Geometry: see drawing. Coordinates: mm, zero at the bounding-box minimum. A direction names the side the tool comes from. Coordinates: 2 decimals unless noted, no trailing zeros. Write each loop counter-clockwise with the first axis right and the second up, starting at its lowest first coordinate (ties: lowest second). Pieces come first, ordered by that corner, then holes. Notation, with made-up numbers: M 75.5,9 L 112.5,9 A32 cw 112.5,44 Z; hole C 68.5,41 d3. An arc over 180 degrees is marked long. Write item = value, one per line. Start each with the question number.
1. Pull-direction query (X, two-part tool) for the marked faces 3 and 4; classes: pulls with the +X half, pulls with the -X half, needs draft (parallel to the pull), parting line crosses it, or undercut.
2. Section query A-A (y = 15). Output: boundary loops of the cut face in (x, z).
3. Access query for the marked faces 1 and 2. Directions: +Z, -Z, +X, -X, +Y, -Y. A direction counts if a zero-diameter tool reaches every point of the face in a straight line with its end or side. Return the directions, or none.
4. Section query B-B (z = 24). Output: boundary loops of the cut face in (x, y), then the cut area to 3 significant figures.
5. Section query C-C (x = 49). Output: boundary loops of the cut face in (y, z).
6. Section query D-D (z = 47.5). Output: boundary loops of the cut face in (x, y).
7. Line query: line 1 along X through (y, z) = (16.5, 8); line 2 along Y through (x, z) = (75, 20); line 3 along Z through (x, y) = (63.5, 2). Output: solid intervals per line, ascending.
8. Pin query (flat end, axial travel): pin 1 Ø1.5 at (x, y) = (6, 21) entering from +Z; pin 2 Ø6 at (x, z) = (29.5, 41) entering from -Y; pin 3 Ø1.5 at (x, y) = (72, 20.5) entering from -Z. Return the tip coordinate at first contact, or that it passes through.
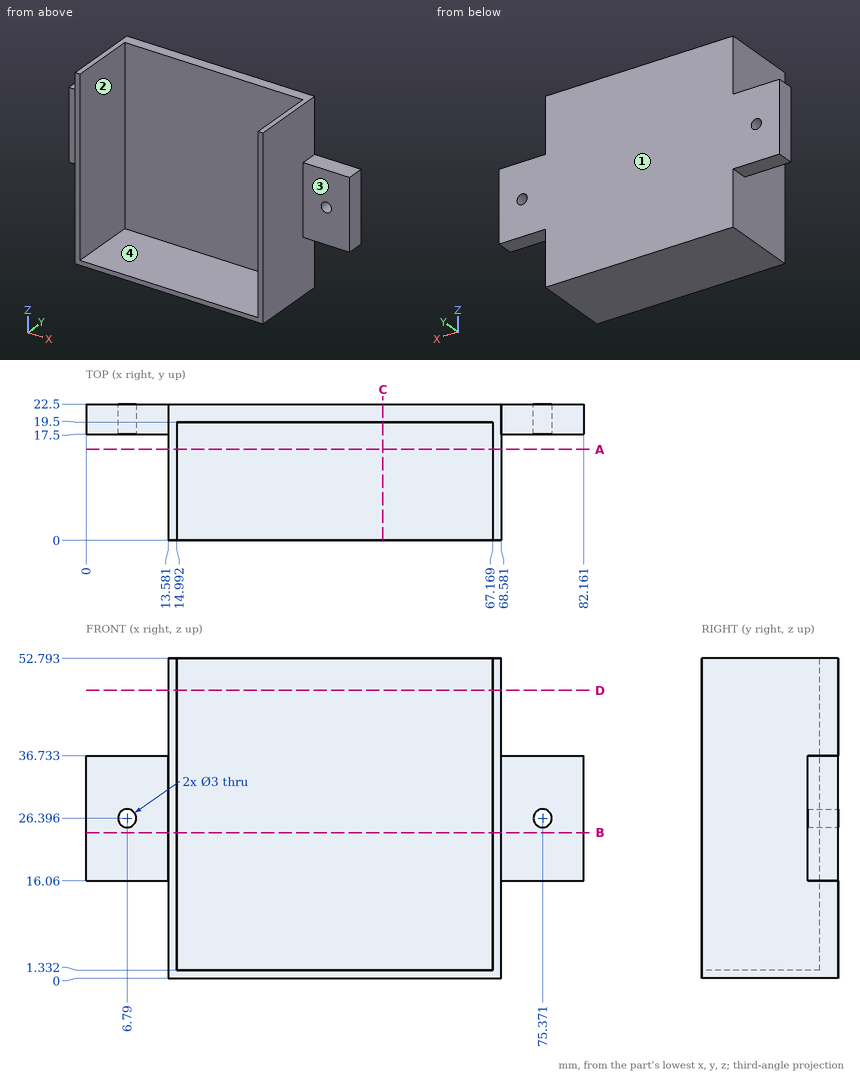
Results are:
q1.face_3 = needs draft
q1.face_4 = undercut
q2.outline = M 13.58,0 L 68.58,0 L 68.58,52.79 L 67.17,52.79 L 67.17,1.33 L 14.99,1.33 L 14.99,52.79 L 13.58,52.79 Z
q3.face_1 = +Z, -Z, +X, -X, +Y
q3.face_2 = +Z, -Y
q4.outline = M 0,17.5 L 13.58,17.5 L 13.58,0 L 14.99,0 L 14.99,19.5 L 67.17,19.5 L 67.17,0 L 68.58,0 L 68.58,17.5 L 82.16,17.5 L 82.16,22.5 L 0,22.5 Z
q4.area = 356 mm^2
q5.outline = M 0,0 L 22.5,0 L 22.5,52.79 L 19.5,52.79 L 19.5,1.33 L 0,1.33 Z
q6.outline = M 13.58,0 L 14.99,0 L 14.99,19.5 L 67.17,19.5 L 67.17,0 L 68.58,0 L 68.58,22.5 L 13.58,22.5 Z
q7.line_1 = 13.58 to 14.99, 67.17 to 68.58
q7.line_2 = 17.5 to 22.5
q7.line_3 = 0 to 1.33
q8.pin_1 = 36.73
q8.pin_2 = 19.5
q8.pin_3 = 16.06
